Can you work these out from the model? Positions are in its coordinate system, mm. Give positions to 0.01 mm unless a question says otherwise; leave off trailing zeros. Write each loop counter-clockwise with the first axis right and the second up, starting at its lowest first coordinate (ties: lowest second). Pieces come first, ordered by that corner, then holes.
from build123d import *

# Parameters (mm, degrees)
SKETCH1_W                             = 425
SKETCH1_H                             = 228.6
BASE_DEPTH                            = 6.35
HOLE_FOR_1_4_BLIND_FASTENERS_B_BS_1_D = 8.7376
HOLE_FOR_1_4_BLIND_FASTENERS_B_BS_2_D = 8.7376


with BuildPart() as part:
    # Sketch1 → Base (new body)
    with BuildSketch(Plane(origin=(0, 0, 0), x_dir=(1, 0, 0), z_dir=(0, 1, 0))):
        with Locations((212.5, -114.3)):
            Rectangle(SKETCH1_W, SKETCH1_H)
    extrude(amount=-BASE_DEPTH)

    # Hole for 1/4 Blind Fasteners (B,BS)1 (through all)
    with Locations(Plane(origin=(0, 0, 0), x_dir=(1, 0, 0), z_dir=(0, 1, 0))):
        with Locations((35.5, -114.3), (125.49982, -114.3), (215.49964, -114.3), (305.49946, -114.3), (395.49928, -114.3)):
            Hole(HOLE_FOR_1_4_BLIND_FASTENERS_B_BS_1_D / 2)

    # Hole for 1/4 Blind Fasteners (B,BS)2 (through all)
    with Locations(Plane(origin=(0, 0, 0), x_dir=(1, 0, 0), z_dir=(0, 1, 0))):
        with Locations((19.05, -19.05), (19.03407818, -208.365498456), (405.95, -19.05), (405.95, -209.55)):
            Hole(HOLE_FOR_1_4_BLIND_FASTENERS_B_BS_2_D / 2)


solid = part.part
(1) Imagine slicing it at C-C, the plane x = 35.5. Write out the boundary of the cut face in (y, z).
Returned:
outline: (-6.35, 0) - (0, 0) - (0, 109.93) - (-6.35, 109.93) - close; (-6.35, 118.67) - (0, 118.67) - (0, 228.6) - (-6.35, 228.6) - close
(2) If we mould it in two halves opening along Z, with no side actions, what happens to faces 1 (the face through (16.701, -3.219, 15.366)), 2 (the face through (210, 0, 113)), 3 (the face through (410.315, -3.219, 209.358))? For each: +Z half, -Z half, draft (parallel to the pull), parting line (faces both ways), or undercut.
Returned:
face 1: undercut
face 2: draft
face 3: undercut
(3) Will this pin go through, and if not, where does the flat tip stop? P1, Ø7, axis at x = 35.5, z = 114.3, coming from the -Y side.
Returned:
P1: passes through
(4) Imagine slicing it at A-A, the plane x = 405.95. Write out the boundary of the cut face in (y, z), plus the area to 3 significant figures.
Returned:
outline: (-6.35, 0) - (0, 0) - (0, 14.68) - (-6.35, 14.68) - close; (-6.35, 23.42) - (0, 23.42) - (0, 205.18) - (-6.35, 205.18) - close; (-6.35, 213.92) - (0, 213.92) - (0, 228.6) - (-6.35, 228.6) - close
area: 1,340 mm2
(5) Imagine slicing it at D-D, the plane z = 19.05. Write out the boundary of the cut face in (x, y).
Returned:
outline: (0, -6.35) - (14.68, -6.35) - (14.68, 0) - (0, 0) - close; (23.42, -6.35) - (401.58, -6.35) - (401.58, 0) - (23.42, 0) - close; (410.32, -6.35) - (425, -6.35) - (425, 0) - (410.32, 0) - close
(6) If I drill on L1, parallel to X at y = -3.25, z = 114.3; L2, parallel to Z at x = 405.95, y = -2.25; L3, parallel to Z at x = 23, y = -3.5, over which ranges is the centre line in solid material (lowest first)?
Returned:
L1: x = 0 to 31.13, 39.87 to 121.13, 129.87 to 211.13, 219.87 to 301.13, 309.87 to 391.13, 399.87 to 425
L2: z = 0 to 14.68, 23.42 to 205.18, 213.92 to 228.6
L3: z = 0 to 17.18, 20.92 to 206.53, 210.2 to 228.6
(7) Imagine slicing it at B-B, the plane z = 114.3. Write out the boundary of the cut face in (x, y), plus the area to 3 significant figures.
Returned:
outline: (0, -6.35) - (31.13, -6.35) - (31.13, 0) - (0, 0) - close; (39.87, -6.35) - (121.13, -6.35) - (121.13, 0) - (39.87, 0) - close; (129.87, -6.35) - (211.13, -6.35) - (211.13, 0) - (129.87, 0) - close; (219.87, -6.35) - (301.13, -6.35) - (301.13, 0) - (219.87, 0) - close; (309.87, -6.35) - (391.13, -6.35) - (391.13, 0) - (309.87, 0) - close; (399.87, -6.35) - (425, -6.35) - (425, 0) - (399.87, 0) - close
area: 2,420 mm2
